CAD build for the part. Positions are in the model's coordinates, mm. A direction names the side the tool comes from. Coordinates: 2 decimals unless noted, no trailing zeros. Write each loop counter-clockwise with the first axis right and the second up, starting at its lowest first coordinate (ties: lowest second). Pieces come first, ordered by that corner, then holes. Notation, with made-up numbers: (10, 69.5) - (44, 69.5) arc R6 ccw to (44, 78.5) - close; hole circle Ø4 at (26, 57.5). An arc over 180 degrees is marked (long way). One line per question, with ' | ' between items. Start each with the question number.
1. Flat gauge pins, fed straight in: P1, Ø2.5, axis at y = 4, z = 0, coming from the +X side; P2, Ø1.5, axis at x = 2, y = 6.5, coming from the +Z side; P3, Ø2, axis at x = 3, y = 13.5, coming from the +Z side. Where does each tip first touch, or does it go through?
2. Which spindle directions (+Z, -Z, +X, -X, +Y, -Y) get a long thin tool onto all of the face, cutting with end or side? Do faces 4 (the flat face through (-1.3, 12, 5.5)), 5 (the cylindrical face through (1.847, 8.874, -0.766)), 6 (the cylindrical face through (-4.761, 5.386, 0.575)). Say none if no direction does.
3. Band-saw the part on D-D, the plane x = 4. Write the cut outline in (y, z).
4. Band-saw the part on C-C, the plane x = -2.25. Write the cut outline in (y, z).
5. Band-saw the part on B-B, the plane z = 0. Write the cut outline in (x, y).
6. Probe line 1 (X direction, y = 12.5, z = 0); line 2 (X direction, y = 17, z = -1.5); line 3 (Z direction, x = -1, y = 10.75). List the from-to ranges inside material, lowest first.
7. Two-plate mould, pull along Z, no slides. Class faces 1 (the flat face through (-2.97, 14.96, -5.04)), 2 (the flat face through (5.85, 15, 0)), 3 (the cylindrical face through (-3, 2.64, 0.06)): +Z half, -Z half, draft (parallel to the pull), parting line (faces both ways), or undercut.
Autodesk Inventor part; units mm, degrees
ref_plane "工作平面2" through (-5.5, 0, 0) normal (1, 0, 0) x (0, 1, 0)
ref_plane "XZ Plane" through (0, 0, 0) normal (0, 1, 0) x (-1, 0, 0)
ref_plane "XY Plane" through (0, 0, 0) normal (0, 0, 1) x (1, 0, 0)
sketch "草圖1" plane through (0, 0, 0) normal (0, 1, 0) x (-1, 0, 0)
  circle A0 centre (0, 0) radius 5.5
  dimension "d0" = 11
extrude "擠出1" add sketch "草圖1" along normal blind 12
sketch "草圖2" plane through (0, 12, 0) normal (0, 1, 0) x (1, 0, 0)
  line L0 (5.85, -3.3775) -> (0, -6.755)
  line L1 (0, -6.755) -> (-5.85, -3.3775)
  line L2 (-5.85, -3.3775) -> (-5.85, 3.3775)
  line L3 (-5.85, 3.3775) -> (0, 6.755)
  line L4 (0, 6.755) -> (5.85, 3.3775)
  line L5 (5.85, 3.3775) -> (5.85, -3.3775)
  point P0 (0, 0)
  point P1 (0, 0)
  dimension "d3" = 11.7
extrude "擠出2" add sketch "草圖2" along normal blind 6
sketch "草圖3" plane through (0, 0, 0) normal (0, -1, 0) x (1, 0, 0)
  circle A0 centre (0, 0) radius 2
  dimension "d6" = 4
extrude "擠出3" cut sketch "草圖3" against normal up to surface (18 mm away)
sketch "草圖5" plane through (0, 0, 0) normal (1, 0, 0) x (0, 1, 0)
  circle A0 centre (4, 0) radius 1.361
  point P0 (0, 0)
  dimension "d12" = 4
extrude "擠出5" cut sketch "草圖5" against normal through all
sketch "草圖6" plane through (0, 0, 0) normal (0, -1, 0) x (1, 0, 0)
  circle A0 centre (0, 0) radius 2
  circle A1 centre (0, 0) radius 5.5
  circle A2 centre (0, 0) radius 2
  line L0 (1.0536, 1.7) -> (-1.0536, 1.7)
  dimension "d15" = 1.7
ref_plane "工作平面2" through (-5.5, 0, 0) normal (1, 0, 0) x (0, 1, 0)
ref_plane "工作平面1" through (5.5, 0, 0) normal (1, 0, 0) x (0, 1, 0)
sketch "草圖7" plane through (-5.5, 0, 0) normal (1, 0, 0) x (0, 1, 0)
  spline S0 degree 5 poles (5.361, 0) (5.361, 0.1236) (5.347, 0.2463) (5.3194, 0.3649) (5.2798, 0.4768) (5.1704, 0.7094) (5.0945, 0.8261) (5.0077, 0.929) (4.9122, 1.0182) (4.67, 1.1972) (4.517, 1.2762) (4.3518, 1.3325) (4.1759, 1.361) (3.8245, 1.361) (3.6486, 1.3326) (3.4837, 1.2765) (3.3306, 1.1975) (3.1182, 1.0408) (3.0486, 0.98) (2.9834, 0.9125) (2.9233, 0.8382) (2.7861, 0.6333) (2.7171, 0.4936) (2.6652, 0.3374) (2.639, 0.1686) (2.639, -0.1236) (2.653, -0.2463) (2.6806, -0.3649) (2.7202, -0.4768) (2.8296, -0.7094) (2.9055, -0.8261) (2.9923, -0.929) (3.0878, -1.0182) (3.33, -1.1972) (3.483, -1.2762) (3.6482, -1.3325) (3.8241, -1.361) (4.1755, -1.361) (4.3514, -1.3326) (4.5163, -1.2765) (4.6694, -1.1975) (4.9141, -1.0169) (5.0116, -0.9254) (5.1001, -0.8195) (5.177, -0.6991) (5.2842, -0.4643) (5.3217, -0.355) (5.3478, -0.2394) (5.361, -0.1201) (5.361, 0) knots 0 0 0 0 0 0 0.063036 0.063036 0.063036 0.063036 0.142762 0.142762 0.142762 0.142762 0.249982 0.249982 0.249982 0.249982 0.35698 0.35698 0.35698 0.35698 0.413527 0.413527 0.413527 0.413527 0.499667 0.499667 0.499667 0.499667 0.562796 0.562796 0.562796 0.562796 0.64264 0.64264 0.64264 0.64264 0.750018 0.750018 0.750018 0.750018 0.857175 0.857175 0.857175 0.857175 0.93874 0.93874 0.93874 0.93874 1 1 1 1 1 1
  circle A0 centre (4, 0) radius 1.5
  point P0 (0, 0)
  dimension "d17" = 3
extrude "擠出6" cut sketch "草圖7" along normal blind 1.5
properties part number "Coupling"
Filled in:
1) P1: stops at x = 5.5 | P2: stops at z = 5.36 | P3: stops at z = 5.6
2) face 4: -Y | face 5: +Y, -Y | face 6: -X
3) outline: (0, -3.77) - (12, -3.77) - (12, -4.45) - (18, -4.45) - (18, 4.45) - (12, 4.45) - (12, 3.77) - (0, 3.77) - close
4) outline: (0, -5.02) - (12, -5.02) - (12, -5.46) - (18, -5.46) - (18, 5.46) - (12, 5.46) - (12, 5.02) - (0, 5.02) - close; hole circle Ø2.72 at (4, 0)
5) outline: (-5.85, 12) - (-5.5, 12) - (-5.5, 5.5) - (-4, 5.5) - (-4, 5.36) - (-2, 5.36) - (-2, 18) - (-5.85, 18) - close; (-5.5, 0) - (-2, 0) - (-2, 2.64) - (-4, 2.64) - (-4, 2.5) - (-5.5, 2.5) - close; (2, 0) - (5.5, 0) - (5.5, 12) - (5.85, 12) - (5.85, 18) - (2, 18) - close
6) line 1: x = -5.85 to -2, 2 to 5.85 | line 2: x = -5.85 to -1.32, 1.32 to 5.85 | line 3: z = -5.41 to -1.73, 1.73 to 5.41
7) face 1: -Z half | face 2: draft | face 3: undercut
